```python
from build123d import *

# Parameters (mm, degrees)
IZIM1_R                     = 13.95
Y_KSEKLIK_EKSTR_ZYON1_DEPTH = 10.6
PAH1_SIZE                   = 4
PAH1_SIZE2                  = 2.5
IZIM3_R                     = 2.5
KES_EKSTR_ZYON1_DEPTH       = 10.6
KES_EKSTR_ZYON2_DEPTH       = 3.6
DAIRESEL_KAPLAMA1_COUNT     = 8
KES_EKSTR_ZYON3_DEPTH       = 10.1


with BuildPart() as part:
    # Çizim1 → Yükseklik-Ekstrüzyon1 (new body)
    with BuildSketch(Plane.XY):
        Circle(IZIM1_R)
    extrude(amount=Y_KSEKLIK_EKSTR_ZYON1_DEPTH)

    # Pah1
    pah1_edges = [part.edges().sort_by_distance(p)[0] for p in [
        (-13.95, 0, 0),
    ]]
    pah1_side = [part.faces().sort_by_distance(p)[0] for p in [
        (0, 0, 0),
    ]]
    chamfer(pah1_edges, length=PAH1_SIZE, length2=PAH1_SIZE2, reference=pah1_side[0])

    # Çizim3 → Kes-Ekstrüzyon1 (cut)
    with BuildSketch(Plane.XY.offset(10.6)):
        Circle(IZIM3_R)
    extrude(amount=-KES_EKSTR_ZYON1_DEPTH, mode=Mode.SUBTRACT)

    # Çizim5 → Kes-Ekstrüzyon2 (cut)
    with BuildSketch(Plane(origin=(0, 0, 0), x_dir=(-1, 0, 0), z_dir=(0, 0, -1))):
        with BuildLine():
            Line((-9.374663228, 3.334394903), (-13.143372063, 4.674855165))
            ThreePointArc((-13.143372063, 4.674855165), (-13.95, 0), (-13.143372063, -4.674855165))
            Line((-13.143372063, -4.674855165), (-9.374663228, -3.334394903))
            ThreePointArc((-9.374663228, -3.334394903), (-9.95, 0), (-9.374663228, 3.334394903))
        make_face()
    kes_ekstr_zyon2 = extrude(amount=-KES_EKSTR_ZYON2_DEPTH, mode=Mode.SUBTRACT)

    # Dairesel Kaplama1: Kes-Ekstrüzyon2 ×8 about axis
    dairesel_kaplama1_axis = Axis((0, 0, 0), (0, 0, 1))
    for i in range(1, DAIRESEL_KAPLAMA1_COUNT):
        add(kes_ekstr_zyon2.rotate(dairesel_kaplama1_axis, i * 360 / DAIRESEL_KAPLAMA1_COUNT), mode=Mode.SUBTRACT)

    # Çizim8 → Kes-Ekstrüzyon3 (cut)
    with BuildSketch(Plane(origin=(0, 0, 0.5), x_dir=(-1, 0, 0), z_dir=(0, 0, -1))):
        with BuildLine():
            ThreePointArc((-9.374663228, -3.334394903), (-9.192601348, -3.807700152), (-8.986661187, -4.271114693))
            ThreePointArc((-8.986661187, -4.271114693), (-7.035712473, -7.035712473), (-4.271114693, -8.986661187))
            ThreePointArc((-4.271114693, -8.986661187), (-3.807700152, -9.192601348), (-3.334394903, -9.374663228))
            ThreePointArc((-3.334394903, -9.374663228), (0, -9.95), (3.334394903, -9.374663228))
            ThreePointArc((3.334394903, -9.374663228), (3.807700152, -9.192601348), (4.271114693, -8.986661187))
            ThreePointArc((4.271114693, -8.986661187), (7.035712473, -7.035712473), (8.986661187, -4.271114693))
            ThreePointArc((8.986661187, -4.271114693), (9.192601348, -3.807700152), (9.374663228, -3.334394903))
            ThreePointArc((9.374663228, -3.334394903), (9.95, 0), (9.374663228, 3.334394903))
            ThreePointArc((9.374663228, 3.334394903), (9.192601348, 3.807700152), (8.986661187, 4.271114693))
            ThreePointArc((8.986661187, 4.271114693), (7.035712473, 7.035712473), (4.271114693, 8.986661187))
            ThreePointArc((4.271114693, 8.986661187), (3.807700152, 9.192601348), (3.334394903, 9.374663228))
            ThreePointArc((3.334394903, 9.374663228), (0, 9.95), (-3.334394903, 9.374663228))
            ThreePointArc((-3.334394903, 9.374663228), (-3.807700152, 9.192601348), (-4.271114693, 8.986661187))
            ThreePointArc((-4.271114693, 8.986661187), (-7.035712473, 7.035712473), (-8.986661187, 4.271114693))
            ThreePointArc((-8.986661187, 4.271114693), (-9.192601348, 3.807700152), (-9.374663228, 3.334394903))
            ThreePointArc((-9.374663228, 3.334394903), (-9.95, 0), (-9.374663228, -3.334394903))
        make_face()
    extrude(amount=-KES_EKSTR_ZYON3_DEPTH, mode=Mode.SUBTRACT)


solid = part.part
```
Part model, mm, in its own coordinate system. A direction names the side the tool comes from. Round coordinates to 2 decimals unless told otherwise and drop trailing zeros. Loops run counter-clockwise (first coordinate to the right, second up) from the corner with the lowest first, then second, coordinate; pieces in that order, holes last. Notation, with made-up numbers: (30, 84) -> (89, 84) arc R16 cw to (89, 90) -> close; hole circle Ø2 at (47.5, -19.5). An arc over 180 degrees is marked (long way). Use one line per item in the form item = value. Start each with the question number.
Item 1: Drill centre lines: line 1 along Y through (x, z) = (0, 0.45); line 2 along Z through (x, y) = (-9.5, -5); line 3 along X through (y, z) = (0, 4). Where is each one in solid material? Low to high.
Item 2: Band-saw the part on A-A (z = 4.75). List the corners of the cut face in (x, y).
Item 3: Two-plate mould, pull along X, no slides. Class faces 6 (the conical face through (-4.592, -11.063, 1.267)), 7 (the flat face through (-12, 0, 3.6)), 8 (the flat face through (-3.846, 10.814, 2.175)): released by +X, released by -X, zero draft, split by the parting line, or undercut.
Item 4: Band-saw the part on D-D (y = -5.5). Give the number of separate pieces and of enclosed holes in the cut face, plus the area to 3 significant figures.
Item 5: Tool access for faces 1 (the flat face through (-2, -2, 0.5)), 2 (the conical face through (-4.58, 11.07, 1.27)), 3 (the flat face through (4.93, 10.37, 2.17)), 4 (the flat face through (-10.814, -3.846, 2.175)), 5 (the flat face through (3.846, -10.814, 2.175)): list every direction of +Z, -Z, +X, -X, +Y, -Y with a clear straight run to the whole face (end or side of a thin tool).
Item 6: Band-saw the part on B-B (x = 0). List the corners of the cut face in (y, z), plus the area to 4 significant figures.
Item 7: Drop flat-ended pins along their axis: pin 1 Ø12 at (x, y) = (-2, -10.5) entering from -Z; pin 2 Ø2.5 at (x, y) = (12.5, 0) entering from -Z; pin 3 Ø4 at (y, z) = (4, 6) entering from -X; pin 4 Ø1 at (x, z) = (-10.5, 3.5) entering from +Y. Give the stop position or say it passes through.
Data:
q1.line_1 = -9.95 to -2.5, 2.5 to 9.95
q1.line_2 = 3.6 to 10.6
q1.line_3 = -13.95 to -9.95, 9.95 to 13.95
q2.outline = circle Ø27.9 at (0, 0); hole (-4.27, 8.99) arc R9.95 ccw to (4.27, -8.99) arc R9.95 ccw to start
q3.face_6 = released by -X
q3.face_7 = zero draft
q3.face_8 = undercut
q4.separate_pieces = 3
q4.enclosed_holes = 0
q4.area = 75.3 mm^2
q5.face_1 = +Z
q5.face_2 = -Z, -X, +Y
q5.face_3 = -Z, +X
q5.face_4 = -Z, -X
q5.face_5 = -Z, -Y
q6.outline = (-13.95, 3.6) -> (-9.95, 3.6) -> (-9.95, 10.6) -> (-13.95, 10.6) -> close; (-9.95, 0) -> (-2.5, 0) -> (-2.5, 0.5) -> (-9.95, 0.5) -> close; (2.5, 0) -> (9.95, 0) -> (9.95, 0.5) -> (2.5, 0.5) -> close; (9.95, 3.6) -> (13.95, 3.6) -> (13.95, 10.6) -> (9.95, 10.6) -> close
q6.area = 63.45 mm^2
q7.pin_1 = 0
q7.pin_2 = 3.6
q7.pin_3 = -13.81
q7.pin_4 = 9.72
